from build123d import *

# Parameters (mm, degrees)
SKETCH2_W           = 18
SKETCH2_H           = 24
SKETCH2_R           = 1.25
BOSS_EXTRUDE2_DEPTH = 2
SKETCH3_W           = 18
SKETCH3_H           = 2
BOSS_EXTRUDE3_DEPTH = 21
SKETCH4_W           = 18
SKETCH4_H           = 2.5
BOSS_EXTRUDE4_DEPTH = 26
SKETCH5_W           = 18
SKETCH5_H           = 3
BOSS_EXTRUDE5_DEPTH = 42.5
SKETCH15_R          = 1
CUT_EXTRUDE3_DEPTH  = 2


with BuildPart() as part:
    # Sketch2 → Boss-Extrude2 (new body)
    with BuildSketch(Plane(origin=(0, 0, 0), x_dir=(1, 0, 0), z_dir=(0, 1, 0))):
        with Locations((-11, 4)):
            Rectangle(SKETCH2_W, SKETCH2_H)
        with Locations(Location((-17, -6, 0), (0, 0, 270))):
            Circle(SKETCH2_R, mode=Mode.SUBTRACT)
        with Locations(Location((-17, -2, 0), (0, 0, 270))):
            Circle(SKETCH2_R, mode=Mode.SUBTRACT)
        with Locations(Location((-17, 2, 0), (0, 0, 270))):
            Circle(SKETCH2_R, mode=Mode.SUBTRACT)
        with Locations(Location((-17, 6, 0), (0, 0, 270))):
            Circle(SKETCH2_R, mode=Mode.SUBTRACT)
        with Locations(Location((-17, 10, 0), (0, 0, 270))):
            Circle(SKETCH2_R, mode=Mode.SUBTRACT)
        with Locations(Location((-17, 14, 0), (0, 0, 270))):
            Circle(SKETCH2_R, mode=Mode.SUBTRACT)
        with Locations(Location((-13, -4, 0), (0, 0, 270))):
            Circle(SKETCH2_R, mode=Mode.SUBTRACT)
        with Locations(Location((-13, 0, 0), (0, 0, 270))):
            Circle(SKETCH2_R, mode=Mode.SUBTRACT)
        with Locations(Location((-13, 4, 0), (0, 0, 270))):
            Circle(SKETCH2_R, mode=Mode.SUBTRACT)
        with Locations(Location((-13, 8, 0), (0, 0, 270))):
            Circle(SKETCH2_R, mode=Mode.SUBTRACT)
        with Locations(Location((-13, 12, 0), (0, 0, 270))):
            Circle(SKETCH2_R, mode=Mode.SUBTRACT)
        with Locations(Location((-9, -6, 0), (0, 0, 270))):
            Circle(SKETCH2_R, mode=Mode.SUBTRACT)
        with Locations(Location((-9, -2, 0), (0, 0, 270))):
            Circle(SKETCH2_R, mode=Mode.SUBTRACT)
        with Locations(Location((-9, 2, 0), (0, 0, 270))):
            Circle(SKETCH2_R, mode=Mode.SUBTRACT)
        with Locations(Location((-9, 6, 0), (0, 0, 270))):
            Circle(SKETCH2_R, mode=Mode.SUBTRACT)
        with Locations(Location((-9, 10, 0), (0, 0, 270))):
            Circle(SKETCH2_R, mode=Mode.SUBTRACT)
        with Locations(Location((-9, 14, 0), (0, 0, 270))):
            Circle(SKETCH2_R, mode=Mode.SUBTRACT)
        with Locations(Location((-5, -4, 0), (0, 0, 270))):
            Circle(SKETCH2_R, mode=Mode.SUBTRACT)
        with Locations(Location((-5, 0, 0), (0, 0, 270))):
            Circle(SKETCH2_R, mode=Mode.SUBTRACT)
        with Locations(Location((-5, 4, 0), (0, 0, 270))):
            Circle(SKETCH2_R, mode=Mode.SUBTRACT)
        with Locations(Location((-5, 8, 0), (0, 0, 270))):
            Circle(SKETCH2_R, mode=Mode.SUBTRACT)
        with Locations(Location((-5, 12, 0), (0, 0, 270))):
            Circle(SKETCH2_R, mode=Mode.SUBTRACT)
    extrude(amount=BOSS_EXTRUDE2_DEPTH)

    # Sketch3 → Boss-Extrude3 (add)
    with BuildSketch(Plane.XY.offset(8)):
        with Locations((-11, 1)):
            Rectangle(SKETCH3_W, SKETCH3_H)
    extrude(amount=BOSS_EXTRUDE3_DEPTH)

    # Sketch4 → Boss-Extrude4 (add)
    with BuildSketch(Plane(origin=(0, 0, 0), x_dir=(-1, 0, 0), z_dir=(0, -1, 0))):
        with Locations((11, -27.75)):
            Rectangle(SKETCH4_W, SKETCH4_H)
    extrude(amount=BOSS_EXTRUDE4_DEPTH)

    # Sketch5 → Boss-Extrude5 (add)
    with BuildSketch(Plane(origin=(0, 0, 26.5), x_dir=(-1, 0, 0), z_dir=(0, 0, -1))):
        with Locations((11, -24.5)):
            Rectangle(SKETCH5_W, SKETCH5_H)
    extrude(amount=BOSS_EXTRUDE5_DEPTH)

    # Sketch15 → Cut-Extrude3 (cut)
    with BuildSketch(Plane(origin=(0, -23, 0), x_dir=(1, 0, 0), z_dir=(0, 1, 0))):
        with Locations(Location((-17, -6, 0), (0, 0, 270))):
            Circle(SKETCH15_R)
        with Locations(Location((-17, -2, 0), (0, 0, 270))):
            Circle(SKETCH15_R)
        with Locations(Location((-17, 2, 0), (0, 0, 270))):
            Circle(SKETCH15_R)
        with Locations(Location((-17, 6, 0), (0, 0, 270))):
            Circle(SKETCH15_R)
        with Locations(Location((-17, 10, 0), (0, 0, 270))):
            Circle(SKETCH15_R)
        with Locations(Location((-17, 14, 0), (0, 0, 270))):
            Circle(SKETCH15_R)
        with Locations(Location((-13, -4, 0), (0, 0, 270))):
            Circle(SKETCH15_R)
        with Locations(Location((-13, 0, 0), (0, 0, 270))):
            Circle(SKETCH15_R)
        with Locations(Location((-13, 4, 0), (0, 0, 270))):
            Circle(SKETCH15_R)
        with Locations(Location((-13, 8, 0), (0, 0, 270))):
            Circle(SKETCH15_R)
        with Locations(Location((-13, 12, 0), (0, 0, 270))):
            Circle(SKETCH15_R)
        with Locations(Location((-9, -6, 0), (0, 0, 270))):
            Circle(SKETCH15_R)
        with Locations(Location((-9, -2, 0), (0, 0, 270))):
            Circle(SKETCH15_R)
        with Locations(Location((-9, 2, 0), (0, 0, 270))):
            Circle(SKETCH15_R)
        with Locations(Location((-9, 6, 0), (0, 0, 270))):
            Circle(SKETCH15_R)
        with Locations(Location((-9, 10, 0), (0, 0, 270))):
            Circle(SKETCH15_R)
        with Locations(Location((-9, 14, 0), (0, 0, 270))):
            Circle(SKETCH15_R)
        with Locations(Location((-5, -4, 0), (0, 0, 270))):
            Circle(SKETCH15_R)
        with Locations(Location((-5, 0, 0), (0, 0, 270))):
            Circle(SKETCH15_R)
        with Locations(Location((-5, 4, 0), (0, 0, 270))):
            Circle(SKETCH15_R)
        with Locations(Location((-5, 8, 0), (0, 0, 270))):
            Circle(SKETCH15_R)
        with Locations(Location((-5, 12, 0), (0, 0, 270))):
            Circle(SKETCH15_R)
    extrude(amount=-CUT_EXTRUDE3_DEPTH, mode=Mode.SUBTRACT)


solid = part.part
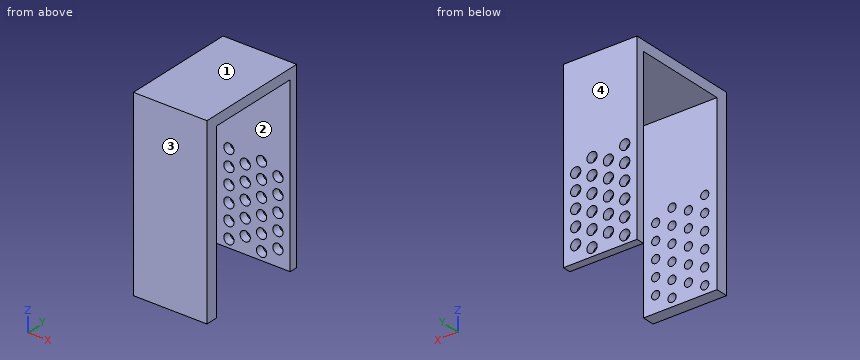
Geometry: final body of the model. Coordinates: model frame, mm. Face numbers are marked on the shaded views. Give positions to 0.01 mm unless a question says otherwise; leave off trailing zeros. Write each loop counter-clockwise with the first axis right and the second up, starting at its lowest first coordinate (ties: lowest second). Pieces come first, ordered by that corner, then holes. Notation, with made-up numbers: (67.25, 54.5) - (86.25, 54.5) arc R19 cw to (86.25, 82.5) - close; hole circle Ø5 at (26.25, 79.25). An arc over 180 degrees is marked (long way). Return JSON: item names as keys, results as strings. Group by question number.
1) Section A-A on z = 13.5. Return the cut outline in (x, y).
2) Section B-B on z = -6. Return the cut outline in (x, y).
3) Mould query, pull axis Y, two halves, no side actions, for the marked faces 1, 2, 3 and 4. Classes: released by +Y, released by -Y, zero draft, split by the parting line, or undercut.
4) First-contact query: P1, Ø1, axis at x = -5, z = -12, coming from the +Y side; P2, Ø10, axis at x = -15, y = -10, coming from the -Z side; P3, Ø10, axis at y = -6, z = -1, coming from the -X side. Flat tips, straight axial feed; report the tip coordinate or a pass-through.
5) Section C-C on x = -9. State how many separate pieces and enclosed holes the cut face has, plus the area to 4 significant figures.
6) Line query: line 1 (X direction, y = 0.9, z = -6); line 2 (X direction, y = -23.45, z = -2); line 3 (Z direction, x = -13.25, y = 1). Output: solid intervals per line, ascending.
Filled in:
{
 "1": {"outline": "(-20, -26) - (-2, -26) - (-2, -23) - (-20, -23) - close; (-20, 0) - (-2, 0) - (-2, 2) - (-20, 2) - close"},
 "2": {"outline": "(-20, -26) - (-2, -26) - (-2, -23) - (-8, -23) - (-8, -25) - (-10, -25) - (-10, -23) - (-16, -23) - (-16, -25) - (-18, -25) - (-18, -23) - (-20, -23) - close; (-20, 0) - (-18.25, 0) - (-18.25, 2) - (-20, 2) - close; (-15.75, 0) - (-10.25, 0) - (-10.25, 2) - (-15.75, 2) - close; (-7.75, 0) - (-2, 0) - (-2, 2) - (-7.75, 2) - close"},
 "3": {"face 1": "zero draft", "face 2": "undercut", "face 3": "released by -Y", "face 4": "released by +Y"},
 "4": {"P1": "stops at y = -25", "P2": "stops at z = 26.5", "P3": "passes through"},
 "5": {"separate pieces": "7", "enclosed holes": "0", "area": "228.5 mm^2"},
 "6": {"line 1": "x = -20 to -18.25, -15.75 to -10.25, -7.75 to -2", "line 2": "x = -20 to -18, -16 to -10, -8 to -2", "line 3": "z = -16 to -13.22, -10.78 to -9.22, -6.78 to -5.22, -2.78 to -1.22, 1.22 to 2.78, 5.22 to 29"}
}
